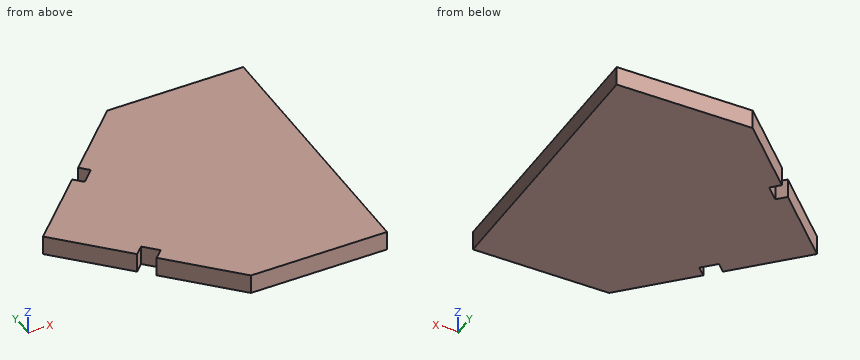
Autodesk Inventor part; units mm, degrees
ref_plane "YZ Plane" through (0, 0, 0) normal (1, 0, 0) x (0, 1, 0)
ref_plane "XZ Plane" through (0, 0, 0) normal (0, 1, 0) x (-1, 0, 0)
ref_plane "XY Plane" through (0, 0, 0) normal (0, 0, 1) x (1, 0, 0)
sketch "Sketch1" plane through (0, 0, 0) normal (0, 0, 1) x (1, 0, 0)
  line L0 (0, 35) -> (35, 35)
  line L1 (35, 35) -> (35, -35)
  line L2 (0, -35) -> (-35, 0)
  line L3 (0, 35) -> (-35, 0)
  line L4 (35, -35) -> (0, -35)
  point P0 (0, 0)
  dimension "d1" = 70
extrude "Extrusion1" add sketch "Sketch1" along normal blind 5
sketch "Sketch2" plane through (0, 0, 5) normal (0, 0, 1) x (1, 0, 0)
  line L0 (0, 35) -> (-35, 0)
  line L1 (-35, 0) -> (0, -35)
  line L2 (-13.7396, 17.0178) -> (-15.8609, 19.1391)
  line L3 (-17.0178, 13.7396) -> (-19.1391, 15.8609)
  line L4 (-13.7396, 17.0178) -> (-17.0178, 13.7396)
  line L5 (0, 0) -> (-35, 0)
  line L6 (-13.7396, -17.0178) -> (-15.8609, -19.1391)
  line L7 (-17.0178, -13.7396) -> (-19.1391, -15.8609)
  line L8 (-13.7396, -17.0178) -> (-17.0178, -13.7396)
  line L9 (-15.8609, 19.1391) -> (-19.1391, 15.8609)
  line L10 (-19.1391, -15.8609) -> (-15.8609, -19.1391)
  dimension "d6" = 4.636
extrude "Extrusion2" cut sketch "Sketch2" against normal blind 5
properties part number "frame1"
Can you work these out from the model? Positions are in its coordinate system, mm. Round coordinates to 2 decimals unless told otherwise and drop trailing zeros. Loops run counter-clockwise (first coordinate to the right, second up) from the corner with the lowest first, then second, coordinate; pieces in that order, holes last. Notation, with made-up numbers: (86, -19.75) - (126, -19.75) arc R37 cw to (126, 17.25) - close; hole circle Ø7 at (-17.75, 78). An arc over 180 degrees is marked (long way). Answer in a Markdown table with one row per item. Add a question column.
Q1. I want a section at A-A on z = 3.25. List the corners of the cut face in (x, y) for me, and give its area (3 significant figures).
Q2. I want a section at C-C on x = -1. List the corners of the cut face in (y, z) for me, and give its area (3 significant figures).
Q3. I want a section at B-B on y = 7. List the corners of the cut face in (x, z) for me, and give its area (3 significant figures).
Q4. I need wall thicknesses on L1, parallel to X at y = 15.5, z = 1.6; L2, parallel to Y at x = -27.5, z = 0.2; L3, parallel to X at y = 27, z = 3.75. Which ranges of each line are inside material? Lowest first, please.
Q5. For pin 1 Ø1.5 at (x, z) = (-20, 2.5) entering from -Y, with a flat end and sliding along its axis, tell me the tip position at first contact or that it passes through.
A:
| question | item | result |
|---|---|---|
| 1 | outline | (-35, 0) - (-19.14, -15.86) - (-17.02, -13.74) - (-13.74, -17.02) - (-15.86, -19.14) - (0, -35) - (35, -35) - (35, 35) - (0, 35) - (-15.86, 19.14) - (-13.74, 17.02) - (-17.02, 13.74) - (-19.14, 15.86) - close |
| 1 | area | 3,650 mm^2 |
| 2 | outline | (-34, 0) - (34, 0) - (34, 5) - (-34, 5) - close |
| 2 | area | 340 mm^2 |
| 3 | outline | (-28, 0) - (35, 0) - (35, 5) - (-28, 5) - close |
| 3 | area | 315 mm^2 |
| 4 | L1 | -19.5 to -18.78, -15.26 to 35 |
| 4 | L2 | -7.5 to 7.5 |
| 4 | L3 | -8 to 35 |
| 5 | pin 1 | y = -15.75 |
